```python
from build123d import *

# Parameters (mm, degrees)
SKETCH_1_R      = 15
EXTRUDE_1_DEPTH = 20
SKETCH_2_W      = 5
SKETCH_2_H      = 15


with BuildPart() as part:
    # 草图1 → 凸台-拉伸1 (new body)
    with BuildSketch(Plane(origin=(0, 0, 0), x_dir=(1, 0, 0), z_dir=(0, 1, 0))):
        Circle(SKETCH_1_R)
        with BuildLine():
            Line((1.53, -5.5), (0, -5.5))
            Line((0, -5.5), (-1.5, -5.5))
            Line((-1.5, -5.5), (-1.5, -3.708099244))
            ThreePointArc((-1.5, -3.708099244), (-2.839864336, 2.816943477), (3.695821965, 1.53))
            Line((3.695821965, 1.53), (5.5, 1.53))
            Line((5.5, 1.53), (5.5, 0))
            Line((5.5, 0), (5.5, -1.5))
            Line((5.5, -1.5), (3.708099244, -1.5))
            ThreePointArc((3.708099244, -1.5), (2.839864336, -2.816943477), (1.53, -3.695821965))
            Line((1.53, -3.695821965), (1.53, -5.5))
        make_face(mode=Mode.SUBTRACT)
    extrude(amount=EXTRUDE_1_DEPTH)

    # 草图2 → 切除-旋转1 (revolve, cut)
    with BuildSketch(Plane.XY):
        with Locations((12.5, 9.892021361)):
            Rectangle(SKETCH_2_W, SKETCH_2_H)
    revolve(axis=Axis((0, 0, 0), (0, 1, 0)), mode=Mode.SUBTRACT)


solid = part.part
```
The listing builds one solid part. Answer for the finished solid, in the listing's coordinates (mm). A direction names the side the tool comes from. Coordinates: 2 decimals unless noted, no trailing zeros. Loops run counter-clockwise (first coordinate to the right, second up) from the corner with the lowest first, then second, coordinate; pieces in that order, holes last. Notation, with made-up numbers: (58, 74.25) -> (98, 74.25) arc R23 ccw to (98, 84.25) -> close; hole circle Ø1 at (-15.5, -39). An arc over 180 degrees is marked (long way). Return JSON: item names as keys, results as strings. Group by question number.
(1) Determine the mould class of faces 1 (the cylindrical face through (-2.17, 10, 9.76)), 2 (the flat face through (1.53, 10, 5)), 3 (the flat face through (3, 20, 3)), 4 (the flat face through (-3, 2.392, 10)) for opening direction Y: released by +Y, released by -Y, zero draft, split by the parting line, or undercut.
(2) Given pin 1 Ø3.5 at (x, y) = (0.5, 11) entering from -Z; pin 2 Ø2 at (y, z) = (8, -5) entering from +X; pin 3 Ø0.9 at (x, y) = (4.5, 6.5) entering from +Z, each flat-ended and moving along its own axis, determine where each tip first touches the part or whether it passes through.
(3) A cutting plane is placed at B-B on x = 0. Write down the section's boundary in (y, z), and give its area (3 significant figures).
(4) Which of the six approach directions +Z, -Z, +X, -X, +Y, -Y give full straight-line access (tool end or side, diameter ignored) to faces 5 (the flat face through (-1.5, 10, 5)), 6 (the flat face through (3, 0, 3)), 7 (the flat face through (-3, 17.392, 10))?
(5) Find the intervals of material crossed by probe 1 along X at (y, z) = (5.25, 0); probe 2 along Y at (x, z) = (-0.75, 11), in increasing order. Write a range as from..to.
(6) A cutting plane is placed at D-D on x = 8.75. Write down the section's boundary in (y, z), and give its area (3 significant figures).
(7) A cutting plane is placed at A-A on y = 12. Write down the section's boundary in (x, z).
(8) A cutting plane is placed at C-C on z = 0. Write down the section's boundary in (x, y), and give its area (3 significant figures).
The answers:
{
 "1": {"face 1": "undercut", "face 2": "zero draft", "face 3": "released by +Y", "face 4": "undercut"},
 "2": {"pin 1": "stops at z = -10", "pin 2": "stops at x = 9.17", "pin 3": "stops at z = 9.14"},
 "3": {"outline": "(0, -15) -> (2.39, -15) -> (2.39, -10) -> (17.39, -10) -> (17.39, -15) -> (20, -15) -> (20, -4) -> (0, -4) -> close; (0, 5.5) -> (20, 5.5) -> (20, 15) -> (17.39, 15) -> (17.39, 10) -> (2.39, 10) -> (2.39, 15) -> (0, 15) -> close", "area": "260 mm^2"},
 "4": {"face 5": "+Y, -Y", "face 6": "+Z, -Z, +X, -X, -Y", "face 7": "none"},
 "5": {"probe 1": "x = -10..-4, 5.5..10", "probe 2": "y = 0..2.39, 17.39..20"},
 "6": {"outline": "(0, -12.18) -> (2.39, -12.18) -> (2.39, -4.84) -> (17.39, -4.84) -> (17.39, -12.18) -> (20, -12.18) -> (20, 12.18) -> (17.39, 12.18) -> (17.39, 4.84) -> (2.39, 4.84) -> (2.39, 12.18) -> (0, 12.18) -> close", "area": "267 mm^2"},
 "7": {"outline": "circle Ø20 at (0, 0); hole (-1.5, 3.71) arc R4 ccw (long way) to (3.7, -1.53) -> (5.5, -1.53) -> (5.5, 1.5) -> (3.71, 1.5) arc R4 ccw to (1.53, 3.7) -> (1.53, 5.5) -> (-1.5, 5.5) -> close"},
 "8": {"outline": "(-15, 0) -> (-4, 0) -> (-4, 20) -> (-15, 20) -> (-15, 17.39) -> (-10, 17.39) -> (-10, 2.39) -> (-15, 2.39) -> close; (5.5, 0) -> (15, 0) -> (15, 2.39) -> (10, 2.39) -> (10, 17.39) -> (15, 17.39) -> (15, 20) -> (5.5, 20) -> close", "area": "260 mm^2"}
}
